from build123d import *

# Parameters (mm, degrees)
SKETCH_1_W          = 10
SKETCH_1_H          = 70
SKETCH_1_R          = 4
EXTRUDE_1_DEPTH     = 60
SKETCH_2_W          = 44.992308415
SKETCH_2_H          = 17.259344539
CUT_EXTRUDE_1_DEPTH = 76.392930627
FILLET_1_R          = 3


with BuildPart() as part:
    # 草图1 → 凸台-拉伸1 (new body)
    with BuildSketch(Plane.XY):
        with Locations((5, -9.543169943)):
            Rectangle(SKETCH_1_W, SKETCH_1_H)
        with Locations((5, -9.543169943)):
            Circle(SKETCH_1_R, mode=Mode.SUBTRACT)
    extrude(amount=EXTRUDE_1_DEPTH)

    # 草图2 → 切除-拉伸1 (cut, through all)
    with BuildSketch(Plane(origin=(10, 0, 0), x_dir=(0, 0, -1), z_dir=(1, 0, 0))):
        with Locations((-29.753893106, -28.924255962)):
            Rectangle(SKETCH_2_W, SKETCH_2_H)
        with Locations((-29.753893106, 9.837916076)):
            Rectangle(SKETCH_2_W, SKETCH_2_H)
    extrude(amount=-CUT_EXTRUDE_1_DEPTH, mode=Mode.SUBTRACT)

    # 圆角1
    fillet_1_edges = [part.edges().sort_by_distance(p)[0] for p in [
        (5, -44.543169943, 60),
        (10, -28.924255962, 52.250047313),
        (10, -20.294583692, 29.753893106),
        (0, -28.924255962, 7.257738898),
        (0, -37.553928231, 29.753893106),
        (0, -28.924255962, 52.250047313),
        (0, -20.294583692, 29.753893106),
        (10, -37.553928231, 29.753893106),
        (10, -28.924255962, 7.257738898),
        (10, 18.467588345, 29.753893106),
        (10, 9.837916075, 7.257738898),
        (0, 1.208243806, 29.753893106),
        (0, 9.837916075, 52.250047313),
        (0, 18.467588345, 29.753893106),
        (0, 9.837916075, 7.257738898),
        (10, 9.837916075, 52.250047313),
        (10, 1.208243806, 29.753893106),
        (5, 25.456830057, 60),
        (5, -44.543169943, 0),
        (5, 25.456830057, 0),
        (10, 25.456830057, 30),
        (10, -44.543169943, 30),
        (0, -44.543169943, 30),
        (0, 25.456830057, 30),
    ]]
    fillet(fillet_1_edges, radius=FILLET_1_R)


solid = part.part
Design review of the part built by this model. Coordinates are the model's own, in mm. A direction names the side the tool comes from. Round coordinates to 2 decimals unless told otherwise and drop trailing zeros. Order: outer loops, then holes, each group sorted by start corner. A loop starts at its lowest first (then second) coordinate and runs counter-clockwise, first axis right, second up. Notation, with made-up numbers: M 37.5,37 L 61.5,37 A30 ccw 61.5,71 Z; hole C 7.25,17 d2. An arc over 180 degrees is marked long. Answer as CSV lines item,"result". Start each with the question number.
1) Add section A-A (x = 5). Give the boundary of the cut face in (y, z).
2) Add section C-C (z = 31.5). Give the boundary of the cut face in (x, y), then the cut area to 3 significant figures.
3) The part is to be moulded in two halves that separate along Y. For faces 1 (the face through (9.098, 19.323, 29.397)), 2 (the face through (5, -44.543, 30)), 3 (the face through (5, -29, 52.25)), 4 (the face through (5.07, 24.15, 59.476)), say which applies: +Y half, -Y half, draft (parallel to the pull), parting line (faces both ways), or undercut.
4) Wall thickness on line 1 along Y through (x, z) = (5, 39.5); line 2 along Y through (x, z) = (5, 57); line 3 along Y through (x, z) = (2.25, 14.5): over which ranges is each line inside the solid? List them lowest first. Write a range as [from, to].
5) Add section B-B (y = 17). Give the boundary of the cut face in (x, z), then the cut area to 3 significant figures.
6) Add section D-D (z = 6.5). Give the boundary of the cut face in (x, y), then the cut area to 3 significant figures.
7) Tool access review of faces 5 (the face through (5, 10, 7.258)), 6 (the face through (9.1, 10, 53.11)), 7 (the face through (0.86, -29.09, 53.15)), 8 (the face through (9.1, 24.6, 30.4)), 9 (the face through (5.07, 24.15, 0.524)): name each direction out of +Z, -Z, +X, -X, +Y, -Y from which nothing blocks a thin tool from reaching the whole face with its end or side.
Resolved:
1,outline,"M -44.54,3 A3 ccw -41.54,0 L -13.54,0 L -13.54,60 L -41.54,60 A3 ccw -44.54,57 Z; M -5.54,0 L 22.46,0 A3 ccw 25.46,3 L 25.46,57 A3 ccw 22.46,60 L -5.54,60 Z; hole M -37.55,7.26 L -20.29,7.26 L -20.29,52.25 L -37.55,52.25 Z; hole M 1.21,7.26 L 18.47,7.26 L 18.47,52.25 L 1.21,52.25 Z"
2,outline,"M 0,-41.54 A3 ccw 3,-44.54 L 7,-44.54 A3 ccw 10,-41.54 L 10,-40.55 A3 ccw 7,-37.55 L 3,-37.55 A3 ccw 0,-40.55 Z; M 0,-17.29 A3 ccw 3,-20.29 L 7,-20.29 A3 ccw 10,-17.29 L 10,-1.79 A3 ccw 7,1.21 L 3,1.21 A3 ccw 0,-1.79 Z; M 0,21.47 A3 ccw 3,18.47 L 7,18.47 A3 ccw 10,21.47 L 10,22.46 A3 ccw 7,25.46 L 3,25.46 A3 ccw 0,22.46 Z; hole C 5,-9.54 d8"
2,area,"281 mm^2"
3,face 1,"undercut"
3,face 2,"-Y half"
3,face 3,"undercut"
3,face 4,"+Y half"
4,line 1,"[-44.54, -37.55], [-20.29, -13.54], [-5.54, 1.21], [18.47, 25.46]"
4,line 2,"[-44.54, -13.54], [-5.54, 25.46]"
4,line 3,"[-44.45, -37.65], [-20.2, -12.45], [-6.64, 1.11], [18.56, 25.36]"
5,outline,"M 0,0 L 10,0 L 10,4.26 A3 ccw 7,7.26 L 3,7.26 A3 ccw 0,4.26 Z; M 0,55.25 A3 ccw 3,52.25 L 7,52.25 A3 ccw 10,55.25 L 10,60 L 0,60 Z"
5,area,"142 mm^2"
6,outline,"M 0,-41.54 A3 ccw 3,-44.54 L 7,-44.54 A3 ccw 10,-41.54 L 10,-40.55 A3 ccw 8.99,-38.31 L 8.99,-19.54 A3 ccw 10,-17.29 L 10,-1.79 A3 ccw 8.99,0.45 L 8.99,19.23 A3 ccw 10,21.47 L 10,22.46 A3 ccw 7,25.46 L 3,25.46 A3 ccw 0,22.46 L 0,21.47 A3 ccw 1.01,19.23 L 1.01,0.45 A3 ccw 0,-1.79 L 0,-17.29 A3 ccw 1.01,-19.54 L 1.01,-38.31 A3 ccw 0,-40.55 Z; hole C 5,-9.54 d8"
6,area,"561 mm^2"
7,face 5,"+X, -X"
7,face 6,"+X"
7,face 7,"-X"
7,face 8,"+Z, -Z, +X, +Y"
7,face 9,"-Z, +X, -X, +Y"
